For this review, take the finished solid that the model builds, in its own axes (mm). Face numbers are marked on the shaded views. A direction names the side the tool comes from. Round coordinates to 2 decimals unless told otherwise and drop trailing zeros. Order: outer loops, then holes, each group sorted by start corner. A loop starts at its lowest first (then second) coordinate and runs counter-clockwise, first axis right, second up. Notation, with made-up numbers: (-3, 32) -> (39, 32) arc R26 cw to (39, 66) -> close; hole circle Ø11 at (-32, 83). An arc over 180 degrees is marked (long way). Put each result on its own line as item: value. Start each with the question number.
```python
from build123d import *

# Parameters (mm, degrees)
EXTRUDE_1_DEPTH     = 32
SKETCH_3_R          = 4
EXTRUDE_2_DEPTH     = 9
SKETCH_4_R          = 2.5
CUT_EXTRUDE_1_DEPTH = 49.174035829


with BuildPart() as part:
    # 草图2 → 凸台-拉伸1 (new body)
    with BuildSketch(Plane(origin=(0, 0, 0), x_dir=(1, 0, 0), z_dir=(0, 1, 0))):
        with BuildLine():
            Line((-0.620533184, 16.939122741), (-0.620533184, 7.076499426))
            ThreePointArc((-0.620533184, 7.076499426), (-0.865551691, 5.978035603), (-1.554155931, 5.087821563))
            ThreePointArc((-1.554155931, 5.087821563), (-2.634503149, 5.403268433), (-3.47838812, 6.147926068))
            Line((-3.47838812, 6.147926068), (-9.275492654, 14.126955939))
            ThreePointArc((-9.275492654, 14.126955939), (-9.514491938, 14.94638072), (-9.177971495, 15.730811482))
            ThreePointArc((-9.177971495, 15.730811482), (-10.550745279, 14.826476488), (-11.835029396, 13.800345917))
            ThreePointArc((-11.835029396, 13.800345917), (-10.985000873, 13.877993441), (-10.279536436, 13.397475432))
            Line((-10.279536436, 13.397475432), (-4.482431902, 5.41844556))
            ThreePointArc((-4.482431902, 5.41844556), (-4.034995203, 4.385751395), (-4.068833052, 3.260801691))
            ThreePointArc((-4.068833052, 3.260801691), (-5.128267329, 2.880991407), (-6.248683387, 2.987408949))
            Line((-6.248683387, 2.987408949), (-15.62859556, 6.035127162))
            ThreePointArc((-15.62859556, 6.035127162), (-16.303595844, 6.557575481), (-16.49242192, 7.389995052))
            ThreePointArc((-16.49242192, 7.389995052), (-17.071464467, 5.851476488), (-17.507327728, 4.266436154))
            ThreePointArc((-17.507327728, 4.266436154), (-16.865280276, 4.82888855), (-16.012106158, 4.854802907))
            Line((-16.012106158, 4.854802907), (-6.632193986, 1.807084693))
            ThreePointArc((-6.632193986, 1.807084693), (-5.663207692, 1.234614256), (-5.029354242, 0.304621439))
            ThreePointArc((-5.029354242, 0.304621439), (-5.663207692, -0.625371378), (-6.632193986, -1.197841815))
            Line((-6.632193986, -1.197841815), (-16.012106158, -4.245560029))
            ThreePointArc((-16.012106158, -4.245560029), (-16.865280276, -4.219645672), (-17.507327728, -3.657193276))
            ThreePointArc((-17.507327728, -3.657193276), (-17.071464467, -5.24223361), (-16.49242192, -6.780752173))
            ThreePointArc((-16.49242192, -6.780752173), (-16.303595844, -5.948332603), (-15.62859556, -5.425884284))
            Line((-15.62859556, -5.425884284), (-6.248683387, -2.37816607))
            ThreePointArc((-6.248683387, -2.37816607), (-5.128267329, -2.271748529), (-4.068833052, -2.651558813))
            ThreePointArc((-4.068833052, -2.651558813), (-4.034995203, -3.776508517), (-4.482431902, -4.809202682))
            Line((-4.482431902, -4.809202682), (-10.279536436, -12.788232554))
            ThreePointArc((-10.279536436, -12.788232554), (-10.985000873, -13.268750563), (-11.835029396, -13.191103039))
            ThreePointArc((-11.835029396, -13.191103039), (-10.550745279, -14.21723361), (-9.177971495, -15.121568604))
            ThreePointArc((-9.177971495, -15.121568604), (-9.514491938, -14.337137842), (-9.275492654, -13.517713061))
            Line((-9.275492654, -13.517713061), (-3.47838812, -5.53868319))
            ThreePointArc((-3.47838812, -5.53868319), (-2.634503149, -4.794025555), (-1.554155931, -4.478578685))
            ThreePointArc((-1.554155931, -4.478578685), (-0.865551691, -5.368792725), (-0.620533184, -6.467256547))
            Line((-0.620533184, -6.467256547), (-0.620533184, -16.329879863))
            ThreePointArc((-0.620533184, -16.329879863), (-0.908824502, -17.133288691), (-1.642152093, -17.570104755))
            ThreePointArc((-1.642152093, -17.570104755), (0, -17.645378561), (1.642152093, -17.570104755))
            ThreePointArc((1.642152093, -17.570104755), (0.908824502, -17.133288691), (0.620533184, -16.329879863))
            Line((0.620533184, -16.329879863), (0.620533184, -6.467256547))
            ThreePointArc((0.620533184, -6.467256547), (0.865551691, -5.368792725), (1.554155931, -4.478578685))
            ThreePointArc((1.554155931, -4.478578685), (2.634503149, -4.794025555), (3.47838812, -5.53868319))
            Line((3.47838812, -5.53868319), (9.275492654, -13.517713061))
            ThreePointArc((9.275492654, -13.517713061), (9.514491938, -14.337137842), (9.177971495, -15.121568604))
            ThreePointArc((9.177971495, -15.121568604), (10.550745279, -14.21723361), (11.835029396, -13.191103039))
            ThreePointArc((11.835029396, -13.191103039), (10.985000873, -13.268750563), (10.279536436, -12.788232554))
            Line((10.279536436, -12.788232554), (4.482431902, -4.809202682))
            ThreePointArc((4.482431902, -4.809202682), (4.034995203, -3.776508517), (4.068833052, -2.651558813))
            ThreePointArc((4.068833052, -2.651558813), (5.128267329, -2.271748529), (6.248683387, -2.37816607))
            Line((6.248683387, -2.37816607), (15.62859556, -5.425884284))
            ThreePointArc((15.62859556, -5.425884284), (16.303595844, -5.948332603), (16.49242192, -6.780752173))
            ThreePointArc((16.49242192, -6.780752173), (17.071464467, -5.24223361), (17.507327728, -3.657193276))
            ThreePointArc((17.507327728, -3.657193276), (16.865280276, -4.219645672), (16.012106158, -4.245560029))
            Line((16.012106158, -4.245560029), (6.632193986, -1.197841815))
            ThreePointArc((6.632193986, -1.197841815), (5.663207692, -0.625371378), (5.029354242, 0.304621439))
            ThreePointArc((5.029354242, 0.304621439), (5.663207692, 1.234614256), (6.632193986, 1.807084693))
            Line((6.632193986, 1.807084693), (16.012106158, 4.854802907))
            ThreePointArc((16.012106158, 4.854802907), (16.865280276, 4.82888855), (17.507327728, 4.266436154))
            ThreePointArc((17.507327728, 4.266436154), (17.071464467, 5.851476488), (16.49242192, 7.389995052))
            ThreePointArc((16.49242192, 7.389995052), (16.303595844, 6.557575481), (15.62859556, 6.035127162))
            Line((15.62859556, 6.035127162), (6.248683387, 2.987408949))
            ThreePointArc((6.248683387, 2.987408949), (5.128267329, 2.880991407), (4.068833052, 3.260801691))
            ThreePointArc((4.068833052, 3.260801691), (4.034995203, 4.385751395), (4.482431902, 5.41844556))
            Line((4.482431902, 5.41844556), (10.279536436, 13.397475432))
            ThreePointArc((10.279536436, 13.397475432), (10.985000873, 13.877993441), (11.835029396, 13.800345917))
            ThreePointArc((11.835029396, 13.800345917), (10.550745279, 14.826476488), (9.177971495, 15.730811482))
            ThreePointArc((9.177971495, 15.730811482), (9.514491938, 14.94638072), (9.275492654, 14.126955939))
            Line((9.275492654, 14.126955939), (3.47838812, 6.147926068))
            ThreePointArc((3.47838812, 6.147926068), (2.634503149, 5.403268433), (1.554155931, 5.087821563))
            ThreePointArc((1.554155931, 5.087821563), (0.865551691, 5.978035603), (0.620533184, 7.076499426))
            Line((0.620533184, 7.076499426), (0.620533184, 16.939122741))
            ThreePointArc((0.620533184, 16.939122741), (0.908824502, 17.742531569), (1.642152093, 18.179347633))
            ThreePointArc((1.642152093, 18.179347633), (0, 18.254621439), (-1.642152093, 18.179347633))
            ThreePointArc((-1.642152093, 18.179347633), (-0.908824502, 17.742531569), (-0.620533184, 16.939122741))
        make_face()
    extrude(amount=EXTRUDE_1_DEPTH)

    # 草图3 → 凸台-拉伸2 (add)
    with BuildSketch(Plane(origin=(0, 32, 0), x_dir=(1, 0, 0), z_dir=(0, 1, 0))):
        with Locations(Location((0, 0, 0), (0, 0, 270))):
            Circle(SKETCH_3_R)
    extrude(amount=EXTRUDE_2_DEPTH)

    # 草图4 → 切除-拉伸1 (cut, through all)
    with BuildSketch(Plane(origin=(0, 41, 0), x_dir=(1, 0, 0), z_dir=(0, 1, 0))):
        with Locations(Location((0, 0, 0), (0, 0, 270))):
            Circle(SKETCH_4_R)
    extrude(amount=-CUT_EXTRUDE_1_DEPTH, mode=Mode.SUBTRACT)


solid = part.part
```
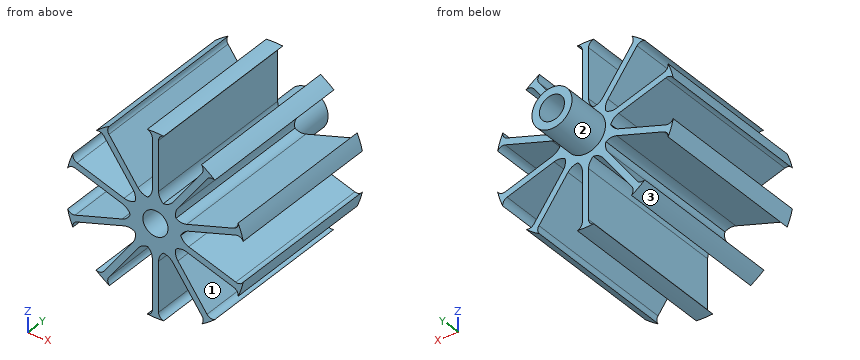
Item 1: Insertion check: pin 1 Ø4 at (x, z) = (0, 0) entering from +Y; pin 2 Ø11 at (y, z) = (14, 9) entering from -X; pin 3 Ø8 at (x, z) = (8, 3.5) entering from +Y; pin 4 Ø4 at (y, z) = (30, 12.5) entering from +X (3 decimals). Each pin has a flat end and moves straight along its axis. Give the tip position at first contact, or say it passes through.
Item 2: Consider section D-D, the plane x = 7.5. Write out the cut boundary in (y, z).
Item 3: Consider section A-A, the plane x = 0. Write out the cut boundary in (y, z).
Item 4: For L1, parallel to Z at x = 11, y = 7; L2, parallel to X at y = 24, z = 8; L3, parallel to X at y = 23, z = -14.5, list the stretches that pass through material, from the lowest coordinate up.
Item 5: Consider section C-C, the plane z = 0.5. Write out the cut boundary in (x, y), plus the area to 3 significant figures.
Item 6: Tool access review of the marked faces 1, 2 and 3: name each direction out of +Z, -Z, +X, -X, +Y, -Y from which nothing blocks a thin tool from reaching the whole face with its end or side.
Item 7: Consider section B-B, the plane z = -9.5. Write out the cut boundary in (x, y), plus the area to 3 significant figures.
Evaluation:
1. pin 1: passes through
1. pin 2: stops at x = -17.51
1. pin 3: stops at y = 32
1. pin 4: stops at x = 11.835
2. outline: (0, -11.68) -> (32, -11.68) -> (32, -9.57) -> (0, -9.57) -> close; (0, -3.39) -> (32, -3.39) -> (32, -2.09) -> (0, -2.09) -> close; (0, 1.48) -> (32, 1.48) -> (32, 2.78) -> (0, 2.78) -> close; (0, 8.96) -> (32, 8.96) -> (32, 11.07) -> (0, 11.07) -> close
3. outline: (0, -18.25) -> (32, -18.25) -> (32, -4) -> (41, -4) -> (41, -2.5) -> (0, -2.5) -> close; (0, 2.5) -> (41, 2.5) -> (41, 4) -> (32, 4) -> (32, 17.65) -> (0, 17.65) -> close
4. L1: z = -14.49 to -13.88, -4.53 to -3.23, 2.62 to 3.92, 13.27 to 13.88
4. L2: x = -6.8 to -5.27, -0.62 to 0.62, 5.27 to 6.8
4. L3: x = -10.99 to -9.46, -0.62 to 0.62, 9.46 to 10.99
5. outline: (-5.54, 0) -> (-2.45, 0) -> (-2.45, 41) -> (-3.97, 41) -> (-3.97, 32) -> (-5.54, 32) -> close; (2.45, 0) -> (5.54, 0) -> (5.54, 32) -> (3.97, 32) -> (3.97, 41) -> (2.45, 41) -> close
5. area: 225 mm^2
6. face 1: +Y, -Y
6. face 2: +Y
6. face 3: -Z, -X, +Y, -Y
7. outline: (-7.45, 0) -> (-5.91, 0) -> (-5.91, 32) -> (-7.45, 32) -> close; (-0.62, 0) -> (0.62, 0) -> (0.62, 32) -> (-0.62, 32) -> close; (5.91, 0) -> (7.45, 0) -> (7.45, 32) -> (5.91, 32) -> close
7. area: 138 mm^2
